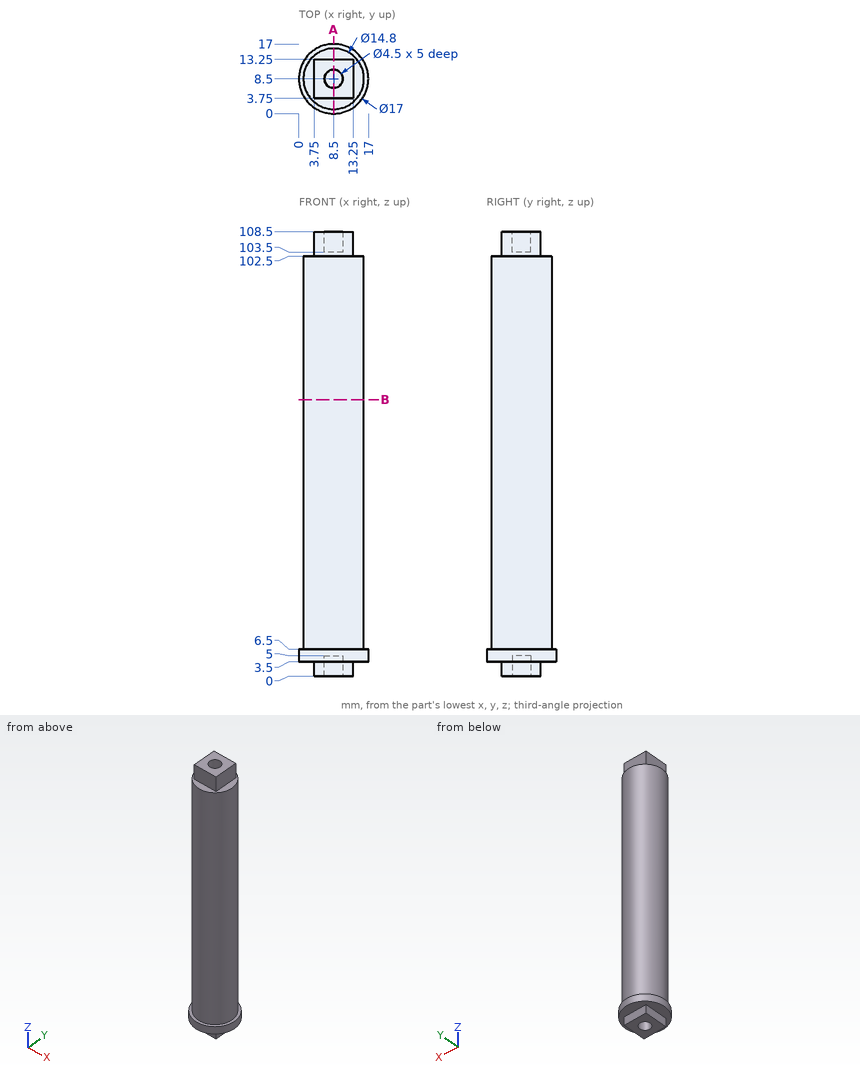
Verification items for this drawing (mm, ordinates from the low corner). Give positions to 0.01 mm unless a question says otherwise; leave off trailing zeros. Write each loop counter-clockwise with the first axis right and the second up, starting at its lowest first coordinate (ties: lowest second). Pieces come first, ordered by that corner, then holes. Notation, with made-up numbers: (87.5, -22) -> (105.5, -22) arc R11 cw to (105.5, -10) -> close; hole circle Ø7 at (-8.75, -1.75). An arc over 180 degrees is marked (long way). Use CSV: the item, a comma, the result in double quotes.
(1) Go/stop test with flat-tipped pins: pin 1 (1.5 mm diameter, centred on y = 6, z = 55, fed in from -X); pin 2 (8 mm diameter, centred on x = 14, z = 95.5, fed in from +Y); pin 3 (4 mm diameter, centred on x = 15, z = 18, fed in from +Y). Record where each tip stops, or that it passes through.
Derived:
pin 1,"stops at x = 1.31"
pin 2,"stops at y = 15.75"
pin 3,"stops at y = 14.37"
(2) Sectioned sample at B-B (z = 67.5). Record the cut outline in (x, y), plus the area to 3 significant figures.
Derived:
outline,"circle Ø14.8 at (8.5, 8.5)"
area,"172 mm^2"
(3) Sectioned sample at A-A (x = 8.5). Record the cut outline in (y, z).
Derived:
outline,"(0, 3.5) -> (3.75, 3.5) -> (3.75, 0) -> (6.25, 0) -> (6.25, 5) -> (10.75, 5) -> (10.75, 0) -> (13.25, 0) -> (13.25, 3.5) -> (17, 3.5) -> (17, 6.5) -> (15.9, 6.5) -> (15.9, 102.5) -> (13.25, 102.5) -> (13.25, 108.5) -> (10.75, 108.5) -> (10.75, 103.5) -> (6.25, 103.5) -> (6.25, 108.5) -> (3.75, 108.5) -> (3.75, 102.5) -> (1.1, 102.5) -> (1.1, 6.5) -> (0, 6.5) -> close"
(4) Material ranges on L1, parallel to Y at x = 8.5, z = 2.3; L2, parallel to Z at x = 16.5, y = 11; L3, parallel to Z at x = 15.5, y = 9.75, recorded low to high.
Derived:
L1,"y = 3.75 to 6.25, 10.75 to 13.25"
L2,"z = 3.5 to 6.5"
L3,"z = 3.5 to 102.5"
